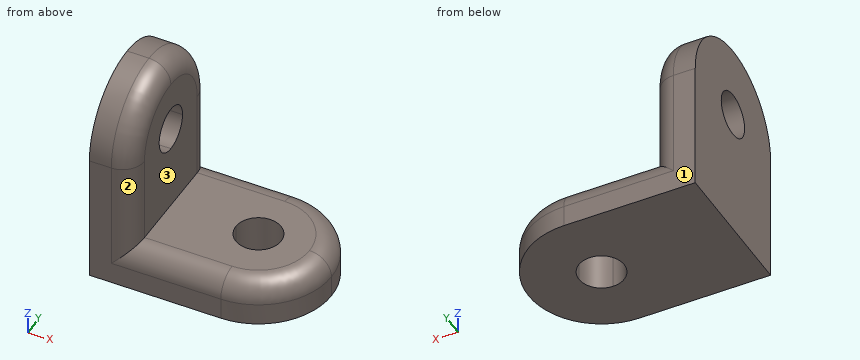
from build123d import *

# Parameters (mm, degrees)
F0_W     = 3
F0_H     = 5
F1_DEPTH = 3
F2_W     = 3
F2_H     = 10
F3_DEPTH = 11
F5_DEPTH = 25
F6_R     = 4.99999
F7_R     = 1.5


# Not quite as in the source:
# - a fillet or chamfer is up to 0.001 mm smaller than in the source, because OpenCascade refuses the exact size


with BuildPart() as f1:
    # F0 (on Top) → F1 (new body)
    with BuildSketch(Plane.XY):
        with Locations((-6.4029270411, -0.9220428518)):
            Rectangle(F0_W, F0_H)
        with Locations((-6.4029270411, -5.9220428518)):
            Rectangle(F0_W, F0_H)
        with BuildLine():
            Line((-4.9029270411, 1.5779571482), (-4.9029270411, -3.4220428518))
            Line((-4.9029270411, -3.4220428518), (-0.4529270411, -3.4220428518))
            ThreePointArc((-0.4529270411, -3.4220428518), (1.0970729589, -1.8720428518), (2.6470729589, -3.4220428518))
            ThreePointArc((2.6470729589, -3.4220428518), (2.1930884698, -4.5180583627), (1.0970729589, -4.9720428518))
            Line((1.0970729589, -4.9720428518), (1.0970729589, -8.4220428518))
            ThreePointArc((1.0970729589, -8.4220428518), (4.6326068649, -6.9575767578), (6.0970729589, -3.4220428518))
            ThreePointArc((6.0970729589, -3.4220428518), (4.6326068649, 0.1134910541), (1.0970729589, 1.5779571482))
            Line((1.0970729589, 1.5779571482), (-4.9029270411, 1.5779571482))
        make_face()
        with BuildLine():
            Line((-0.4529270411, -3.4220428518), (-4.9029270411, -3.4220428518))
            Line((-4.9029270411, -3.4220428518), (-4.9029270411, -8.4220428518))
            Line((-4.9029270411, -8.4220428518), (1.0970729589, -8.4220428518))
            Line((1.0970729589, -8.4220428518), (1.0970729589, -4.9720428518))
            ThreePointArc((1.0970729589, -4.9720428518), (0.0010574481, -4.5180583627), (-0.4529270411, -3.4220428518))
        make_face()
    extrude(amount=F1_DEPTH)

    # F2 (on face) → F3 (join)
    with BuildSketch(Plane.XY.offset(3)):
        with Locations((-6.4029270411, -3.4220428518)):
            Rectangle(F2_W, F2_H)
    extrude(amount=F3_DEPTH)

    # F4 (on face) → F5 (cut)
    with BuildSketch(Plane.YZ.offset(-4.9029270411)):
        with BuildLine():
            ThreePointArc((-1.8720428518, 9), (-4.5180583627, 10.0960155108), (-3.4220428518, 7.45))
            Line((-3.4220428518, 7.45), (-3.4220428518, 9))
            Line((-3.4220428518, 9), (-1.8720428518, 9))
        make_face()
        with BuildLine():
            Line((-3.4220428518, 9), (-3.4220428518, 7.45))
            ThreePointArc((-3.4220428518, 7.45), (-2.326027341, 7.9039844892), (-1.8720428518, 9))
            Line((-1.8720428518, 9), (-3.4220428518, 9))
        make_face()
    extrude(amount=-F5_DEPTH, mode=Mode.SUBTRACT)

    # F6 (radius 5 in the source; OpenCascade refuses exactly that, so slightly less here)
    f6_edges = [f1.edges().sort_by_distance(p)[0] for p in [
        (-6.402927, -8.422043, 14),
        (-6.402927, 1.577957, 14),
    ]]
    fillet(f6_edges, radius=F6_R)

    # F7
    f7_edges = [f1.edges().sort_by_distance(p)[0] for p in [
        (-4.902927, -6.95758, 12.535537),
        (-4.902927, -8.422043, 6.000005),
        (-1.902927, -8.422043, 3),
    ]]
    fillet(f7_edges, radius=F7_R)


solid = f1.part
The listing builds one solid part. Answer for the finished solid, in the listing's coordinates (mm). Face numbers are marked on the shaded views. A direction names the side the tool comes from. Give positions to 0.01 mm unless a question says otherwise; leave off trailing zeros. Order: outer loops, then holes, each group sorted by start corner. A loop starts at its lowest first (then second) coordinate and runs counter-clockwise, first axis right, second up. Notation, with made-up numbers: (-20.5, -10) - (-8.5, -10) arc R21 ccw to (-8.5, 17) - close; hole circle Ø4 at (-25, 6.5). An arc over 180 degrees is marked (long way). Answer as CSV lines item,"result".
Q1. A cutting plane is placed at B-B, the plane y = -2.5. Count the separate pieces of the cut face and the enclosed holes in it, and give its area (3 significant figures).
Answer key:
separate pieces,"3"
enclosed holes,"0"
area,"58.5 mm^2"
Q2. Straight lines are drawn through the part: L1, parallel to Y at x = -7, z = 9; L2, parallel to X at y = -6.75, z = 8; L3, parallel to Z at x = 4.25, y = -3.5. For each, find the intervals that lie inside material, in ascending order.
Answer key:
L1,"y = -8.42 to -4.97, -1.87 to 1.58"
L2,"x = -7.9 to -4.9"
L3,"z = 0 to 3"
Q3. Which of the six approach directions +Z, -Z, +X, -X, +Y, -Y give full straight-line access (tool end or side, diameter ignored) to the marked faces 1, 2 and 3?
Answer key:
face 1,"+Z, -Z, +X, -X, +Y"
face 2,"+Z, +X, -Y"
face 3,"+Z, +X, +Y, -Y"
Q4. Each of these flat-tipped pins is pushed along its axis until it touches: pin 1 Ø3.5 at (y, z) = (-2.5, 7.5) entering from +X; pin 2 Ø2 at (x, y) = (-3, -1.5) entering from +Z. Where does it stop, or does it pass through?
Answer key:
pin 1,"stops at x = -4.9"
pin 2,"stops at z = 3"
Q5. A cutting plane is placed at A-A, the plane x = -2.5. Determine the outline of the cut face in (y, z), and give its area (3 significant figures).
Answer key:
outline,"(-8.42, 0) - (1.58, 0) - (1.58, 1.5) arc R1.5 ccw to (0.08, 3) - (-6.92, 3) arc R1.5 ccw to (-8.42, 1.5) - close"
area,"29.0 mm^2"
